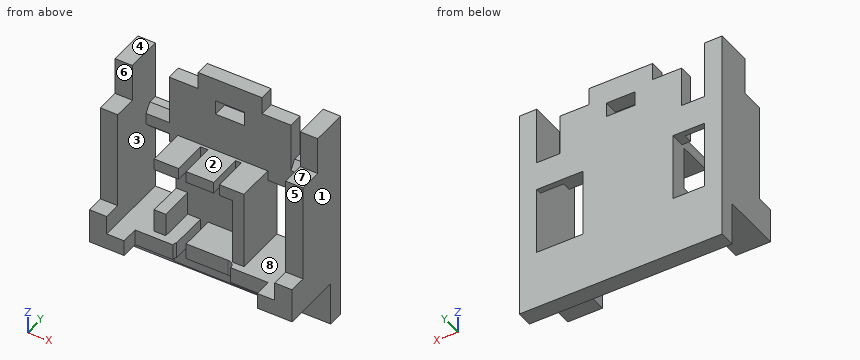
from build123d import *

# Parameters (mm, degrees)
BOSS_EXTRUDE1_DEPTH  = 20.5
SKETCH2_W            = 6
SKETCH2_H            = 13
CUT_EXTRUDE1_DEPTH   = 8
SKETCH3_W            = 23
SKETCH3_H            = 23
BOSS_EXTRUDE2_DEPTH  = 6
BOSS_EXTRUDE4_DEPTH  = 18
SKETCH5_W            = 2.6
SKETCH5_H            = 5.5
SKETCH5_H_2          = 4
SKETCH5_W_2          = 4
SKETCH5_H_3          = 15
SKETCH5_W_3          = 2
CUT_EXTRUDE2_DEPTH   = 14.5
SKETCH9_W            = 70
SKETCH9_H            = 5.5
BOSS_EXTRUDE6_DEPTH  = 15
BOSS_EXTRUDE7_DEPTH  = 7.5
CUT_EXTRUDE3_DEPTH   = 5.5
BOSS_EXTRUDE8_DEPTH  = 6
BOSS_EXTRUDE10_START = -6
BOSS_EXTRUDE10_DEPTH = 58
BOSS_EXTRUDE11_START = -14
SKETCH15_W           = 10
SKETCH15_H           = 5
BOSS_EXTRUDE11_DEPTH = 42
SKETCH16_W           = 42
SKETCH16_H           = 5
BOSS_EXTRUDE12_DEPTH = 20
CUT_EXTRUDE4_REACH   = 28.5
SKETCH17_W           = 10
SKETCH17_H           = 6
SKETCH17_H_2         = 5


with BuildPart() as part:
    # Sketch1 → Boss-Extrude1 (new body)
    with BuildSketch(Plane(origin=(0, 0, 0), x_dir=(1, 0, 0), z_dir=(0, 1, 0))):
        Polygon((29, -29.5), (35, -29.5), (35, 29.5), (-35, 29.5), (-35, -29.5), (-29, -29.5), (-29, 24), (29, 24), align=None)
    extrude(amount=BOSS_EXTRUDE1_DEPTH)

    # Sketch2 → Cut-Extrude1 (cut)
    with BuildSketch(Plane.XZ):
        with Locations((32, 23)):
            Rectangle(SKETCH2_W, SKETCH2_H)
        with Locations((-32, 23)):
            Rectangle(SKETCH2_W, SKETCH2_H)
    extrude(amount=-CUT_EXTRUDE1_DEPTH, mode=Mode.SUBTRACT)



with BuildPart() as body_2:
    # Sketch3 → Boss-Extrude2 (new body)
    with BuildSketch(Plane(origin=(0, 20.5, 0), x_dir=(1, 0, 0), z_dir=(0, 1, 0))):
        with Locations((-2.5, 12.5)):
            Rectangle(SKETCH3_W, SKETCH3_H)
    extrude(amount=-BOSS_EXTRUDE2_DEPTH)


with BuildPart() as part_1:
    add(part.part)

    add(body_2.part)  # Boss-Extrude4 merges body 2
    # Sketch4 → Boss-Extrude4 (add)
    with BuildSketch(Plane(origin=(0, 20.5, 0), x_dir=(1, 0, 0), z_dir=(0, 1, 0))):
        Polygon((-14, 24), (-18, 24), (-18, -3), (13, -3), (13, 24), (9, 24), (9, 1), (-14, 1), align=None)
    extrude(amount=-BOSS_EXTRUDE4_DEPTH)

    # Sketch5 → Cut-Extrude2 (cut)
    with BuildSketch(Plane.XZ):
        with Locations((-8.25, -26.75)):
            Rectangle(SKETCH5_W, SKETCH5_H)
        with Locations((-8.25, 1)):
            Rectangle(SKETCH5_W, SKETCH5_H_2)
        with Locations((-16, -8.5)):
            Rectangle(SKETCH5_W_2, SKETCH5_H_3)
        with Locations((3.55, 1)):
            Rectangle(SKETCH5_W_3, SKETCH5_H_2)
    extrude(amount=-CUT_EXTRUDE2_DEPTH, mode=Mode.SUBTRACT)

    # Sketch9 → Boss-Extrude6 (add)
    with BuildSketch(Plane(origin=(0, 0, -29.5), x_dir=(-1, 0, 0), z_dir=(0, 0, -1))):
        with Locations((0, 17.75)):
            Rectangle(SKETCH9_W, SKETCH9_H)
    extrude(amount=BOSS_EXTRUDE6_DEPTH)

    # Sketch10 → Boss-Extrude7 (add)
    with BuildSketch(Plane.XZ.offset(-15)):
        Polygon((11.5, -29.5), (-11.5, -29.5), (-14.5, -37), (14.5, -37), align=None)
    extrude(amount=BOSS_EXTRUDE7_DEPTH)

    # Sketch11 → Cut-Extrude3 (cut)
    with BuildSketch(Plane(origin=(0, 0, -29.5), x_dir=(-1, 0, 0), z_dir=(0, 0, -1))):
        with BuildLine():
            Line((-7.5, 2.5), (7.5, 2.5))
            ThreePointArc((7.5, 2.5), (10, 0), (7.5, -2.5))
            Line((7.5, -2.5), (-7.5, -2.5))
            ThreePointArc((-7.5, -2.5), (-10, 0), (-7.5, 2.5))
        make_face()
    extrude(amount=-CUT_EXTRUDE3_DEPTH, mode=Mode.SUBTRACT)

    # Sketch12 → Boss-Extrude8 (add)
    with BuildSketch(Plane.XZ):
        Polygon((35, -17.5), (29, -17.5), (29, -24), (23, -24), (23, -29.5), (35, -29.5), align=None)
        Polygon((-23, -24), (-23, -29.5), (-35, -29.5), (-35, -17.5), (-29, -17.5), (-29, -24), align=None)
    extrude(amount=BOSS_EXTRUDE8_DEPTH)

    # Sketch14 → Boss-Extrude10 (add)
    with BuildSketch(Plane(origin=(35, 0, 0), x_dir=(0, 0, -1), z_dir=(1, 0, 0)).offset(BOSS_EXTRUDE10_START)):
        Polygon((-9.5, 20.5), (0.5, 20.5), (0.5, 18.5), (-2.5, 15.5), (-6.5, 15.5), (-9.5, 17.5), align=None)
    extrude(amount=-BOSS_EXTRUDE10_DEPTH)

    # Sketch15 → Boss-Extrude11 (add)
    with BuildSketch(Plane(origin=(35, 0, 0), x_dir=(0, 0, -1), z_dir=(1, 0, 0)).offset(BOSS_EXTRUDE11_START)):
        with Locations((-4.5, 18)):
            Rectangle(SKETCH15_W, SKETCH15_H)
    extrude(amount=-BOSS_EXTRUDE11_DEPTH)

    # Sketch16 → Boss-Extrude12 (add)
    with BuildSketch(Plane.XY.offset(9.5)):
        with Locations((0, 18)):
            Rectangle(SKETCH16_W, SKETCH16_H)
    extrude(amount=BOSS_EXTRUDE12_DEPTH)

    # Sketch17 → Cut-Extrude4 (cut, up to next)
    with BuildSketch(Plane(origin=(0, 20.5, 0), x_dir=(1, 0, 0), z_dir=(0, 1, 0)), mode=Mode.PRIVATE) as cut_extrude4_sk1:
        with Locations((-16, -26.5)):
            Rectangle(SKETCH17_W, SKETCH17_H)
    cut_extrude4_tool1 = extrude(cut_extrude4_sk1.sketch, amount=-CUT_EXTRUDE4_REACH, mode=Mode.PRIVATE) & part_1.part
    add(cut_extrude4_tool1.solids().sort_by_distance((-16, 20.5, 26.5))[0], mode=Mode.SUBTRACT)
    # Sketch17 → Cut-Extrude4 (cut, up to next)
    with BuildSketch(Plane(origin=(0, 20.5, 0), x_dir=(1, 0, 0), z_dir=(0, 1, 0)), mode=Mode.PRIVATE) as cut_extrude4_sk2:
        with Locations((16, -26.5)):
            Rectangle(SKETCH17_W, SKETCH17_H)
    cut_extrude4_tool2 = extrude(cut_extrude4_sk2.sketch, amount=-CUT_EXTRUDE4_REACH, mode=Mode.PRIVATE) & part_1.part
    add(cut_extrude4_tool2.solids().sort_by_distance((16, 20.5, 26.5))[0], mode=Mode.SUBTRACT)
    # Sketch17 → Cut-Extrude4 (cut, up to next)
    with BuildSketch(Plane(origin=(0, 20.5, 0), x_dir=(1, 0, 0), z_dir=(0, 1, 0)), mode=Mode.PRIVATE) as cut_extrude4_sk3:
        with Locations((0, -19)):
            Rectangle(SKETCH17_W, SKETCH17_H_2)
    cut_extrude4_tool3 = extrude(cut_extrude4_sk3.sketch, amount=-CUT_EXTRUDE4_REACH, mode=Mode.PRIVATE) & part_1.part
    add(cut_extrude4_tool3.solids().sort_by_distance((0, 20.5, 19))[0], mode=Mode.SUBTRACT)


solid = part_1.part
The model under review builds one solid part; all positions refer to its coordinate system, in mm. Face numbers are marked on the shaded views. A direction names the side the tool comes from. Round coordinates to 2 decimals unless told otherwise and drop trailing zeros. Loops run counter-clockwise (first coordinate to the right, second up) from the corner with the lowest first, then second, coordinate; pieces in that order, holes last. Notation, with made-up numbers: (-34, 44.5) -> (-19, 44.5) arc R20 ccw to (-19, 54.5) -> close; hole circle Ø8 at (27.5, 68). An arc over 180 degrees is marked (long way). Return JSON: item names as keys, results as strings.
(1) Add section C-C on y = 4.5. State how many separate pieces and enclosed holes the cut face has, plus the area to 3 significant figures.
Solved:
{"separate pieces": "4", "enclosed holes": "0", "area": "1,090 mm2"}
(2) Add section D-D on y = -1.25. Write out the cut boundary in (x, z).
Solved:
{"outline": "(-35, -29.5) -> (-23, -29.5) -> (-23, -24) -> (-29, -24) -> (-29, -17.5) -> (-35, -17.5) -> close; (23, -29.5) -> (35, -29.5) -> (35, -17.5) -> (29, -17.5) -> (29, -24) -> (23, -24) -> close"}
(3) Add section B-B on x = -27.5. Write out the cut boundary in (y, z), plus the area to 3 significant figures.
Solved:
{"outline": "(-6, -29.5) -> (15, -29.5) -> (15, -44.5) -> (20.5, -44.5) -> (20.5, -24) -> (-6, -24) -> close; (15.5, 2.5) -> (18.5, -0.5) -> (20.5, -0.5) -> (20.5, 9.5) -> (17.5, 9.5) -> (15.5, 6.5) -> close", "area": "271 mm2"}
(4) For line 1 (X direction, y = 14.75, z = -5); line 2 (X direction, y = 8.75, z = -7.5); line 3 (Z direction, x = -2, y = 11), list the stretches that pass through material, from the lowest coordinate up.
Solved:
{"line 1": "-35 to -29, -18 to 13, 29 to 35", "line 2": "-35 to -29, 9 to 13, 29 to 35", "line 3": "-37 to -24, -1 to 3"}
(5) The part is to be moulded in two halves that separate along Z. For the marked faces 6, 7 and 8, say which applies: released by +Z, released by -Z, zero draft, split by the parting line, or undercut.
Solved:
{"face 6": "zero draft", "face 7": "released by +Z", "face 8": "undercut"}
(6) For the marked faces 1, 2, 3, 4 and 5, list the 3-axis set-ups (+Z, -Z, +X, -X, +Y, -Y) from which the entire face can be reached by the end or side of a thin tool; tool diameter is ignored.
Solved:
{"face 1": "+Z, -Z, +X, +Y, -Y", "face 2": "+Z, -Y", "face 3": "-Y", "face 4": "+Z, +X, -X, +Y, -Y", "face 5": "+Z, +X, -X, -Y"}
(7) For pin 1 (4.5 mm diameter, centred on x = -15, z = -20, fed in from -Y); pin 2 (6.5 mm diameter, centred on x = 32.5, z = -7.5, fed in from -Y); pin 3 (3 mm diameter, centred on x = 33.5, z = 23.5, fed in from -Y), all flat-tipped, find the tip position at first contact; note any pin that passes through.
Solved:
{"pin 1": "y = 2.5", "pin 2": "y = 0", "pin 3": "y = 8"}
(8) Add section A-A on z = 19. Write out the cut boundary in (x, y), plus the area to 3 significant figures.
Solved:
{"outline": "(-35, 8) -> (-29, 8) -> (-29, 20.5) -> (-35, 20.5) -> close; (-21, 15.5) -> (-5, 15.5) -> (-5, 20.5) -> (-21, 20.5) -> close; (5, 15.5) -> (21, 15.5) -> (21, 20.5) -> (5, 20.5) -> close; (29, 8) -> (35, 8) -> (35, 20.5) -> (29, 20.5) -> close", "area": "310 mm2"}
